For this review, take the finished solid that the model builds, in its own axes (mm). A direction names the side the tool comes from. Round coordinates to 2 decimals unless told otherwise and drop trailing zeros. Order: outer loops, then holes, each group sorted by start corner. A loop starts at its lowest first (then second) coordinate and runs counter-clockwise, first axis right, second up. Notation, with made-up numbers: M 64.25,-16.75 L 108.25,-16.75 A20 cw 108.25,-12.75 Z; hole C 63,-2.75 d9. An arc over 180 degrees is marked long. Put each result on its own line as item: value.
from build123d import *

# Parameters (mm, degrees)
SKETCH2_R           = 53.3
BOSS_EXTRUDE1_DEPTH = 94.62
BOSS_EXTRUDE2_DEPTH = 83
CIRPATTERN1_COUNT   = 13
CIRPATTERN1_ANGLE   = 72
BOSS_EXTRUDE3_START = -40
SKETCH5_R           = 6
BOSS_EXTRUDE3_DEPTH = 70
CIRPATTERN2_COUNT   = 3
CIRPATTERN2_ANGLE   = 180
SKETCH6_R           = 53.3
BOSS_EXTRUDE4_DEPTH = 65.9
FILLET2_R           = 5
SKETCH7_R           = 5
CUT_EXTRUDE1_DEPTH  = 5


with BuildPart() as part:
    # Sketch2 → Boss-Extrude1 (new body)
    with BuildSketch(Plane(origin=(0, 0, 0), x_dir=(0, 0, -1), z_dir=(1, 0, 0))):
        Circle(SKETCH2_R)
    extrude(amount=BOSS_EXTRUDE1_DEPTH)

    # Sketch4 → Boss-Extrude2 (add)
    with BuildSketch(Plane.ZY.offset(-6)):
        Polygon((-0.75, 54.8), (0.75, 54.8), (1.125, 53.288126023), (-1.125, 53.288126023), align=None)
    boss_extrude2 = extrude(amount=-BOSS_EXTRUDE2_DEPTH)

    # CirPattern1: Boss-Extrude2 ×13 about axis
    cirpattern1_axis = Axis((0, 0, 0), (1, 0, 0))
    for i in range(1, CIRPATTERN1_COUNT):
        add(boss_extrude2.rotate(cirpattern1_axis, i * CIRPATTERN1_ANGLE / (CIRPATTERN1_COUNT - 1)))

    # Sketch5 → Boss-Extrude3 (add)
    with BuildSketch(Plane.ZY.offset(-47.31).offset(BOSS_EXTRUDE3_START)):
        with Locations((-57.1, 0)):
            Circle(SKETCH5_R)
    boss_extrude3 = extrude(amount=BOSS_EXTRUDE3_DEPTH)

    # CirPattern2: Boss-Extrude3 ×3 about axis
    cirpattern2_axis = Axis((0, 0, 0), (-1, 0, 0))
    for i in range(1, CIRPATTERN2_COUNT):
        add(boss_extrude3.rotate(cirpattern2_axis, i * CIRPATTERN2_ANGLE / (CIRPATTERN2_COUNT - 1)))

    # Sketch6 → Boss-Extrude4 (add)
    with BuildSketch(Plane(origin=(94.62, 0, 0), x_dir=(0, 0, -1), z_dir=(1, 0, 0))):
        with BuildLine():
            Line((-61.1, 4.472135955), (-27, 63.535068493))
            ThreePointArc((-27, 63.535068493), (-8.298272765, 71.562778811), (4.70027417, 55.902749688))
            ThreePointArc((4.70027417, 55.902749688), (37.380543987, -41.831865022), (-56.077394681, 1.592421361))
            Line((-56.077394681, 1.592421361), (-61.1, 4.472135955))
        make_face()
        Circle(SKETCH6_R, mode=Mode.SUBTRACT)
    extrude(amount=-BOSS_EXTRUDE4_DEPTH)

    # Fillet2
    fillet2_edges = [part.edges().sort_by_distance(p)[0] for p in [
        (61.67, 55.902749688, -4.70027417),
    ]]
    fillet(fillet2_edges, radius=FILLET2_R)

    # Sketch7 → Cut-Extrude1 (cut)
    with BuildSketch(Plane(origin=(94.62, 0, 0), x_dir=(0, 0, -1), z_dir=(1, 0, 0))):
        with Locations((-12.475149036, 27.421809155)):
            Circle(SKETCH7_R)
    extrude(amount=-CUT_EXTRUDE1_DEPTH, mode=Mode.SUBTRACT)


solid = part.part
(1) To check wall thickness, follow L1, parallel to X at y = 45.5, z = 33; L2, parallel to Z at x = 32.5, y = 61; L3, parallel to Z at x = 10.5, y = -2.5. State the ranges of each line that lie inside material, in increasing order.
A:
L1: x = 28.72 to 94.62
L2: z = -3.64 to 28.46
L3: z = -53.24 to 53.24
(2) Add section A-A on z = -17.5. Give the boundary of the cut face in (x, y), then the cut area to 3 significant figures.
A:
outline: M 0,-50.35 L 28.72,-50.35 L 28.72,-53.3 L 94.62,-53.3 L 94.62,53.3 L 28.72,53.3 L 28.72,50.35 L 0,50.35 Z
area: 9,920 mm2
(3) Insertion check: pin 1 Ø4 at (x, y) = (27, 21) entering from -Z; pin 2 Ø0.7 at (y, z) = (46.5, 27) entering from -X; pin 3 Ø8 at (y, z) = (-59.5, 1.5) entering from -X. Each pin has a flat end and moves straight along its axis. Give the tip position at first contact, or say it passes through.
A:
pin 1: stops at z = -52.42
pin 2: stops at x = 6
pin 3: stops at x = 17.31
(4) Draft analysis for pull direction Z (two halves, no side actions). For faces 1 (the face through (0, 1, 1)), 2 (the face through (62.13, 71.91, 10.22)), 3 (the face through (89.62, 27, 13)), 4 (the face through (92.155, 24.379, 16.443)), state which applies: released by +Z, released by -Z, zero draft, split by the parting line, or undercut.
A:
face 1: zero draft
face 2: split by the parting line
face 3: undercut
face 4: undercut
(5) For faces 5 (the face through (62.13, 33.59, 44.29)), 6 (the face through (91.02, 3.01, 58.55)), list the 3-axis set-ups (+Z, -Z, +X, -X, +Y, -Y) from which the entire face can be reached by the end or side of a thin tool; tool diameter is ignored.
A:
face 5: +Z, +X, -X, +Y
face 6: +Z, +X, -Y
(6) Add section B-B on z = -42. Give the boundary of the cut face in (x, y).
A:
outline: M 0,-32.82 L 28.72,-32.82 L 28.72,-37.19 L 94.62,-37.19 L 94.62,37.19 L 28.72,37.19 L 28.72,32.82 L 0,32.82 Z
